CAD build for the part. Positions are in the model's coordinates, mm. Give positions to 0.01 mm unless a question says otherwise; leave off trailing zeros. Order: outer loops, then holes, each group sorted by start corner. A loop starts at its lowest first (then second) coordinate and runs counter-clockwise, first axis right, second up. Notation, with made-up numbers: M 43.25,-14 L 97.25,-14 A14 cw 97.25,1 Z; hole C 53.5,14.5 d10. An arc over 180 degrees is marked long. Put each result on its own line as item: value. Start each with the question number.
1) Cut at D-D (z = 0.75). Give the number of separate pieces and of enclosed holes in the cut face, and give its area (3 significant figures).
2) Cut at C-C (y = 0). Write the cut outline in (x, z).
3) Drill centre lines: line 1 (Y direction, x = 0, z = -0.05); line 2 (Y direction, x = 1.5, z = -0.8); line 3 (X direction, y = 26.5, z = 0.6) (3 decimals). Where is each one in solid material? Low to high. Write a range as [from, to].
4) Cut at B-B (x = -12.7). Write the cut outline in (y, z).
5) Pin check, flat tip, straight feed: pin 1 (6 mm diameter, centred on x = 0, y = 0, fed in from +Z). Stop position of the tip, or through.
6) Cut at A-A (y = 12.7). Write the cut outline in (x, z), and give its area (3 significant figures).
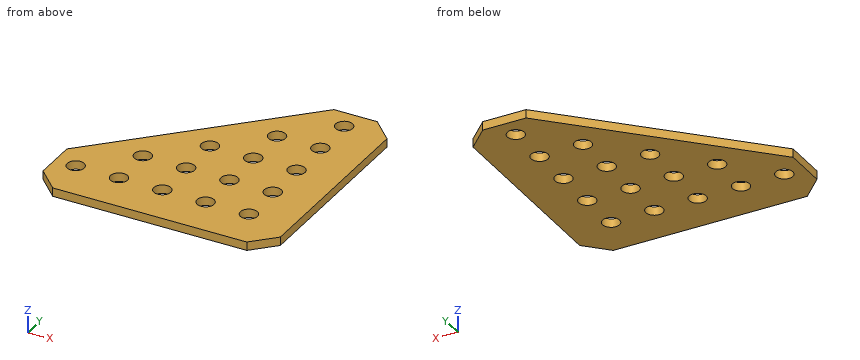
```python
from build123d import *

# Parameters (mm, degrees)
SKETCH1_R           = 2.5
BOSS_EXTRUDE1_DEPTH = 2.5


with BuildPart() as part:
    # Sketch1 → Boss-Extrude1 (new body)
    with BuildSketch(Plane(origin=(0, 0, -1.25), x_dir=(-1, 0, 0), z_dir=(0, 0, -1))):
        Polygon((-6.35, -12.7), (50.546, -12.7), (56.896, -6.35), (56.896, 6.35), (6.35, 56.896), (-6.35, 56.896), (-12.7, 50.546), (-12.7, -6.35), align=None)
        with Locations((0, 12.7)):
            Circle(SKETCH1_R, mode=Mode.SUBTRACT)
        with Locations((0, 25.4)):
            Circle(SKETCH1_R, mode=Mode.SUBTRACT)
        with Locations((12.7, 0)):
            Circle(SKETCH1_R, mode=Mode.SUBTRACT)
        with Locations((25.4, 0)):
            Circle(SKETCH1_R, mode=Mode.SUBTRACT)
        Circle(SKETCH1_R, mode=Mode.SUBTRACT)
        with Locations((50.8, 0)):
            Circle(SKETCH1_R, mode=Mode.SUBTRACT)
        with Locations((38.1, 0)):
            Circle(SKETCH1_R, mode=Mode.SUBTRACT)
        with Locations((0, 50.8)):
            Circle(SKETCH1_R, mode=Mode.SUBTRACT)
        with Locations((0, 38.1)):
            Circle(SKETCH1_R, mode=Mode.SUBTRACT)
        with Locations((12.7, 12.7)):
            Circle(SKETCH1_R, mode=Mode.SUBTRACT)
        with Locations((12.7, 25.4)):
            Circle(SKETCH1_R, mode=Mode.SUBTRACT)
        with Locations((12.7, 38.1)):
            Circle(SKETCH1_R, mode=Mode.SUBTRACT)
        with Locations((25.4, 12.7)):
            Circle(SKETCH1_R, mode=Mode.SUBTRACT)
        with Locations((25.4, 25.4)):
            Circle(SKETCH1_R, mode=Mode.SUBTRACT)
        with Locations((38.1, 12.7)):
            Circle(SKETCH1_R, mode=Mode.SUBTRACT)
    extrude(amount=-BOSS_EXTRUDE1_DEPTH)


solid = part.part
```
Solution:
1. separate pieces: 1
1. enclosed holes: 15
1. area: 3,210 mm²
2. outline: M -56.9,-1.25 L -53.3,-1.25 L -53.3,1.25 L -56.9,1.25 Z; M -48.3,-1.25 L -40.6,-1.25 L -40.6,1.25 L -48.3,1.25 Z; M -35.6,-1.25 L -27.9,-1.25 L -27.9,1.25 L -35.6,1.25 Z; M -22.9,-1.25 L -15.2,-1.25 L -15.2,1.25 L -22.9,1.25 Z; M -10.2,-1.25 L -2.5,-1.25 L -2.5,1.25 L -10.2,1.25 Z; M 2.5,-1.25 L 12.7,-1.25 L 12.7,1.25 L 2.5,1.25 Z
3. line 1: [-12.7, -2.5], [2.5, 10.2], [15.2, 22.9], [27.9, 35.6], [40.6, 48.3], [53.3, 56.9]
3. line 2: [-12.7, -2], [2, 10.7], [14.7, 23.4], [27.4, 36.1], [40.1, 48.8], [52.8, 56.9]
3. line 3: [-36.746, -27.645], [-23.155, -14.945], [-10.455, -2.245], [2.245, 12.7]
4. outline: M -12.7,-1.25 L -2.5,-1.25 L -2.5,1.25 L -12.7,1.25 Z; M 2.5,-1.25 L 10.2,-1.25 L 10.2,1.25 L 2.5,1.25 Z; M 15.2,-1.25 L 22.9,-1.25 L 22.9,1.25 L 15.2,1.25 Z; M 27.9,-1.25 L 35.6,-1.25 L 35.6,1.25 L 27.9,1.25 Z; M 40.6,-1.25 L 50.55,-1.25 L 50.55,1.25 L 40.6,1.25 Z
5. pin 1: z = 1.25
6. outline: M -50.55,-1.25 L -40.6,-1.25 L -40.6,1.25 L -50.55,1.25 Z; M -35.6,-1.25 L -27.9,-1.25 L -27.9,1.25 L -35.6,1.25 Z; M -22.9,-1.25 L -15.2,-1.25 L -15.2,1.25 L -22.9,1.25 Z; M -10.2,-1.25 L -2.5,-1.25 L -2.5,1.25 L -10.2,1.25 Z; M 2.5,-1.25 L 12.7,-1.25 L 12.7,1.25 L 2.5,1.25 Z
6. area: 108 mm²
